```python
from build123d import *

# Parameters (mm, degrees)
SKETCH_1_W          = 50
SKETCH_1_H          = 50
EXTRUDE_1_DEPTH     = 3
SKETCH_2_R          = 5.2
EXTRUDE_3_DEPTH     = 30
SKETCH_4_R          = 4.1
CUT_EXTRUDE_1_DEPTH = 30
CUT_EXTRUDE_2_DEPTH = 30


with BuildPart() as part:
    # 草图1 → 凸台-拉伸1 (new body)
    with BuildSketch(Plane(origin=(0, 0, 0), x_dir=(1, 0, 0), z_dir=(0, 1, 0))):
        with Locations((25, 25)):
            Rectangle(SKETCH_1_W, SKETCH_1_H)
    extrude(amount=EXTRUDE_1_DEPTH)

    # 草图2 → 凸台-拉伸3 (add)
    with BuildSketch(Plane(origin=(0, 3, 0), x_dir=(1, 0, 0), z_dir=(0, 1, 0))):
        with Locations(Location((25, 25, 0), (0, 0, 90))):
            Circle(SKETCH_2_R)
    extrude(amount=EXTRUDE_3_DEPTH)

    # 草图4 → 切除-拉伸1 (cut)
    with BuildSketch(Plane(origin=(0, 33, 0), x_dir=(1, 0, 0), z_dir=(0, 1, 0))):
        with Locations(Location((25, 25, 0), (0, 0, 270))):
            Circle(SKETCH_4_R)
    extrude(amount=-CUT_EXTRUDE_1_DEPTH, mode=Mode.SUBTRACT)

    # 草图6 → 切除-拉伸2 (cut)
    with BuildSketch(Plane.XZ):
        with BuildLine():
            Line((5, -3.25), (45, -3.25))
            ThreePointArc((45, -3.25), (46.75, -5), (45, -6.75))
            Line((45, -6.75), (5, -6.75))
            ThreePointArc((5, -6.75), (3.25, -5), (5, -3.25))
        make_face()
        with BuildLine():
            Line((5, -46.75), (45, -46.75))
            ThreePointArc((45, -46.75), (46.75, -45), (45, -43.25))
            Line((45, -43.25), (5, -43.25))
            ThreePointArc((5, -43.25), (3.25, -45), (5, -46.75))
        make_face()
        with BuildLine():
            Line((6.75, -11.75), (6.75, -38.25))
            ThreePointArc((6.75, -38.25), (5, -40), (3.25, -38.25))
            Line((3.25, -38.25), (3.25, -11.75))
            ThreePointArc((3.25, -11.75), (5, -10), (6.75, -11.75))
        make_face()
        with BuildLine():
            Line((43.25, -11.75), (43.25, -38.25))
            ThreePointArc((43.25, -38.25), (45, -40), (46.75, -38.25))
            Line((46.75, -38.25), (46.75, -11.75))
            ThreePointArc((46.75, -11.75), (45, -10), (43.25, -11.75))
        make_face()
    extrude(amount=-CUT_EXTRUDE_2_DEPTH, mode=Mode.SUBTRACT)


solid = part.part
```
For this review, take the finished solid that the model builds, in its own axes (mm). A direction names the side the tool comes from. Coordinates: 2 decimals unless noted, no trailing zeros. Loops run counter-clockwise (first coordinate to the right, second up) from the corner with the lowest first, then second, coordinate; pieces in that order, holes last. Notation, with made-up numbers: (-13, 22) -> (33, 22) arc R6 cw to (33, 26) -> close; hole circle Ø5 at (51, 36). An arc over 180 degrees is marked (long way). Return JSON: item names as keys, results as strings. Group by question number.
(1) Mouldability with a two-part tool opening along X and no side actions: class faces 4 (the flat face through (25, 1, -50)), 5 (the flat face through (25, 1, -43.25)), 6 (the flat face through (0, 1, -25)) as pulls with the +X half, pulls with the -X half, needs draft (parallel to the pull), parting line crosses it, or undercut.
(2) Consider section D-D, the plane y = 13. Give the boundary of the cut face in (x, z), plus the area to 3 significant figures.
(3) For pin 1 Ø12 at (x, z) = (36.5, -24.5) entering from +Y; pin 2 Ø4 at (x, y) = (29, 14) entering from +Z; pin 3 Ø1.5 at (x, y) = (26.5, 5.5) entering from -Z, all flat-tipped, find the tip position at first contact; note any pin that passes through.
(4) To check wall thickness, follow L1, parallel to X at y = 9, z = -25; L2, parallel to Y at x = 27, z = -23; L3, parallel to X at y = 21.5, z = -26. State the ranges of each line that lie inside material, in increasing order.
(5) Tool access review of faces 1 (the flat face through (46.75, 1, -25)), 2 (the flat face through (25, 1, 0)), 3 (the flat face through (25, 3, -25)): name each direction out of +Z, -Z, +X, -X, +Y, -Y from which nothing blocks a thin tool from reaching the whole face with its end or side.
(6) Consider section A-A, the plane z = -45. Give the boundary of the cut face in (x, y).
(7) Consider section B-B, the plane z = -18. Give the boundary of the cut face in (x, y).
(8) Consider section C-C, the plane x = 40. Give the boundary of the cut face in (y, z).
Results below:
{
 "1": {"face 4": "needs draft", "face 5": "undercut", "face 6": "pulls with the -X half"},
 "2": {"outline": "circle Ø10.4 at (25, -25); hole circle Ø8.2 at (25, -25)", "area": "32.1 mm2"},
 "3": {"pin 1": "stops at y = 3", "pin 2": "stops at z = -20.2", "pin 3": "stops at z = -30.15"},
 "4": {"L1": "x = 19.8 to 20.9, 29.1 to 30.2", "L2": "y = 0 to 3", "L3": "x = 19.9 to 21.02, 28.98 to 30.1"},
 "5": {"face 1": "+Y, -Y", "face 2": "+Z, +X, -X, +Y, -Y", "face 3": "+Y"},
 "6": {"outline": "(0, 0) -> (3.25, 0) -> (3.25, 3) -> (0, 3) -> close; (46.75, 0) -> (50, 0) -> (50, 3) -> (46.75, 3) -> close"},
 "7": {"outline": "(0, 0) -> (3.25, 0) -> (3.25, 3) -> (0, 3) -> close; (6.75, 0) -> (43.25, 0) -> (43.25, 3) -> (6.75, 3) -> close; (46.75, 0) -> (50, 0) -> (50, 3) -> (46.75, 3) -> close"},
 "8": {"outline": "(0, -50) -> (3, -50) -> (3, -46.75) -> (0, -46.75) -> close; (0, -43.25) -> (3, -43.25) -> (3, -6.75) -> (0, -6.75) -> close; (0, -3.25) -> (3, -3.25) -> (3, 0) -> (0, 0) -> close"}
}
